Could you check a few things on this model? Use its own coordinates, in mm. A direction names the side the tool comes from. Round coordinates to 2 decimals unless told otherwise and drop trailing zeros. Loops run counter-clockwise (first coordinate to the right, second up) from the corner with the lowest first, then second, coordinate; pieces in that order, holes last. Notation, with made-up numbers: (37.25, -3.75) - (95.25, -3.75) arc R26 ccw to (95.25, 14.25) - close; hole circle Ø3 at (41.25, 83). An arc over 180 degrees is marked (long way). Use one line per item in the form item = value.
```python
from build123d import *

# Parameters (mm, degrees)
F0_W     = 210
F0_H     = 19.39892
F1_DEPTH = 3
F2_W     = 3
F2_H     = 1.5
F3_DEPTH = 3
F4_W     = 3.5
F4_H     = 2
F5_DEPTH = 4


with BuildPart() as f1:
    # F0 (on Top) → F1 (new body)
    with BuildSketch(Plane.XY):
        Rectangle(F0_W, F0_H)
    extrude(amount=F1_DEPTH)

    # F2 (on face) → F3 (join)
    with BuildSketch(Plane.YZ.offset(105)):
        with Locations((0, 0.75)):
            Rectangle(F2_W, F2_H)
    extrude(amount=F3_DEPTH)

    # F4 (on face) → F5 (cut)
    with BuildSketch(Plane(origin=(-105, 0, 0), x_dir=(0, -1, 0), z_dir=(-1, 0, 0))):
        with Locations((0, 1)):
            Rectangle(F4_W, F4_H)
    extrude(amount=-F5_DEPTH, mode=Mode.SUBTRACT)


solid = f1.part
```
1. For P1, Ø0.9, axis at y = -4.5, z = 1.5, coming from the +X side; P2, Ø1.6, axis at y = -0.5, z = 0.5, coming from the -X side; P3, Ø1.2, axis at x = 106.5, z = 1, coming from the +Y side, each with a flat end and sliding along its axis, tell me the tip position at first contact or that it passes through.
Solution:
P1 = 105
P2 = -101
P3 = 1.5
2. If we section it at A-A, the plane z = 0.7: Write out the boundary of the cut face in (x, y), plus the area to 3 significant figures.
Solution:
outline = (-105, -9.7) - (105, -9.7) - (105, -1.5) - (108, -1.5) - (108, 1.5) - (105, 1.5) - (105, 9.7) - (-105, 9.7) - (-105, 1.75) - (-101, 1.75) - (-101, -1.75) - (-105, -1.75) - close
area = 4,070 mm^2
3. Please list where this line runs through material, in increasing order: line 1 along X through (y, z) = (1.75, 2.3).
Solution:
line_1 = -105 to 105
4. On a 3-axis mill with a long thin cutter (end or side, diameter ignored), from which of +Z, -Z, +X, -X, +Y, -Y can I reach the whole of each face in a straight line? I mean faces 1 (the face through (-1, 0, 3)), 2 (the face through (-103, 0, 2)). Say none if no direction works.
Solution:
face_1 = +Z, +X, -X, +Y, -Y
face_2 = -Z, -X
